Autodesk Inventor part; units mm, degrees
ref_plane "Work Plane1" through (29, 0, 0) normal (0, -1, 0) x (1, 0, 0)
ref_plane "YZ Plane" through (0, 0, 0) normal (1, 0, 0) x (0, 1, 0)
ref_plane "XZ Plane" through (0, 0, 0) normal (0, 1, 0) x (-1, 0, 0)
sketch "Sketch1" plane through (0, 0, 0) normal (0, 0, 1) x (1, 0, 0)
  line L0 (-2.3333, 0) -> (35, 0)
  line L1 (35, 0) -> (35, 5)
  line L2 (35, 5) -> (3.75, 5)
  line L3 (3.75, 5) -> (2.8297, 5)
  line L4 (2.8297, 5) -> (0, 5)
  line L5 (0, 5) -> (0, 8)
  line L6 (0, 8) -> (-10, 8)
  line L7 (-10, 8) -> (-10, 4.6188)
  line L8 (-10, 4.6188) -> (-5, 4.6188)
  line L9 (-5, 4.6188) -> (-2.3333, 0)
  line L10 (-19, 0) -> (44, 0)
  line L11 (0, -1.6) -> (0, 9.6)
  line L12 (3.75, 5) -> (0, 5) construction
  dimension "d1" = 31.25
  dimension "d2" = 0.9203
  dimension "d3" = 10
  dimension "d4" = 5
  dimension "d5" = 60
  dimension "d6" = 10
  dimension "d7" = 10
  dimension "d8" = 9.2376
  dimension "d9" = 16
  dimension "d26" = 35
revolve "Body" add sketch "Sketch1" angle 360 about axis through (-2.3333, 0, 0) along (1, 0, 0)
sketch "Sketch2" plane through (-10, 0, 0) normal (-1, 0, 0) x (0, 0, 1)
  circle A0 centre (0, 0) radius 4.6188
  line L0 (0, -11.2) -> (0, 11.2)
  line L1 (-11.2, 0) -> (11.2, 0)
  line L2 (4.6188, 0) -> (2.3094, -4)
  line L3 (2.3094, -4) -> (-2.3094, -4)
  line L4 (-2.3094, -4) -> (-4.6188, 0)
  line L5 (-4.6188, 0) -> (-2.3094, 4)
  line L6 (-2.3094, 4) -> (2.3094, 4)
  line L7 (2.3094, 4) -> (4.6188, 0)
extrude "Slot" add sketch "Sketch2" against normal up to next contours L7 A0 | A0 L2 | L6 L0 A0 | A0 L0 L3 | L0 L6 A0 | A0 L3 L0 | L4 A0 | A0 L5
fillet "Fillet1" radius 1 1 edges at (-10, -8, 0)
thread "Thread"
chamfer "Chamfer1" distance 0.9202 distance2 0.9202 1 edges at (35, -5, 0) measured on face at (35, 1.974, -0.2121)
ref_plane "Work Plane1" through (29, 0, 0) normal (0, -1, 0) x (1, 0, 0)
fillet "Fillet2" radius 0.1 1 edges at (0, -5, 0)
equation "\"d1\" = GEL"
equation "\"d3\" = KOH"
equation "\"d4\" = INTI"
equation "\"d6\" = GD"
equation "\"d7\" = BDM"
equation "\"d8\" = 1.1547 * SW"
equation "\"d9\" = KOD"
equation "\"d26\" = NLG"
equation "\"d30\" = R"
equation "\"d17\" = RR"
equation "\"d13\" = GEL"
equation "\"d15\" = -0.5 * SPD + 0.5 * GD"
equation "\"d16\" = GUL"
equation "\"GD\" = NND"
equation "\"NLG\" = 35"
equation "\"GEL\" = 31.25"
equation "\"KOD\" = 16"
equation "\"KOH\" = NND"
equation "\"INTI\" = 5"
equation "\"GAL\" = 0.61345 * PTC"
equation "\"GUL\" = 0.61345 * PTC"
equation "\"BDM\" = NND"
equation "\"SW\" = 8"
equation "\"RR\" = 0.1 * NND"
equation "\"SPD\" = NND - 1.2269 * PTC"
equation "\"R\" = 0.1"
equation "\"TOA\" = 30deg"
equation "\"GD1\" = THREADDIA - 1.2269 * PTC"
equation "\"FAWI\" = 45deg"
equation "\"PTC\" = 1.5"
equation "\"E0\" = 1.155 * SW"
properties part number "M10x45 SHCS A2" material "Stainless Steel AISI 304"
Geometry check sheet. Reference: the model listing, model coordinates, mm. A direction names the side the tool comes from. Coordinates: 2 decimals unless noted, no trailing zeros. Loops run counter-clockwise (first coordinate to the right, second up) from the corner with the lowest first, then second, coordinate; pieces in that order, holes last.
Item 1: Access from +Z, -Z, +X, -X, +Y, -Y to the whole of each face (thin tool, end or side, straight path). Record for faces 1 (the face through (0, 5, -2)), 2 (the face through (-7.36, 1.97, -3.48)), 3 (the face through (35, 0, 0)).
Item 2: Release check for a two-part mould opening along Z. For faces 4 (the face through (-10, -5, 0)), 5 (the face through (-2.5, 0.276, -0.087)), 6 (the face through (16.85, -1.08, 4.88)) record: released by +Z, released by -Z, zero draft, split by the parting line, or undercut.
Item 3: Sectioned sample at B-B, the plane x = 19.5. Record the boundary of the cut face in (y, z), then the cut area to 3 significant figures.
Item 4: Thickness scan on line 1 (X direction, y = 4.25, z = -4); line 2 (Z direction, x = -6, y = 3); line 3 (X direction, y = 0.5, z = -2). Record the ranges inside material, lowest first.
Item 5: Sectioned sample at A-A, the plane x = -6. Record the boundary of the cut face in (y, z).
Item 6: Go/stop test with flat-tipped pins: pin 1 Ø2 at (y, z) = (-6, 2.5) entering from +X; pin 2 Ø2 at (x, z) = (8, 2) entering from -Y; pin 3 Ø1 at (x, z) = (-2, 3.5) entering from +Y. Record where each tip stops, or that it passes through.
Check result:
1. face 1: +X
1. face 2: -X
1. face 3: +Z, -Z, +X, +Y, -Y
2. face 4: zero draft
2. face 5: undercut
2. face 6: split by the parting line
3. outline: circle Ø10 at (0, 0)
3. area: 78.5 mm2
4. line 1: x = -10 to 0
4. line 2: z = -7.42 to -2.89, 2.89 to 7.42
4. line 3: x = -3.52 to 35
5. outline: circle Ø16 at (0, 0); hole (-4, -2.31) - (0, -4.62) - (4, -2.31) - (4, 2.31) - (0, 4.62) - (-4, 2.31) - close
6. pin 1: stops at x = 0
6. pin 2: stops at y = -4.9
6. pin 3: stops at y = 7.42
